```python
from build123d import *

# Parameters (mm, degrees)
BOSS_EXTRUDE1_DEPTH = 4
SKETCH3_R           = 2.1
CUT_EXTRUDE1_DEPTH  = 4
CHAMFER1_SIZE       = 3


with BuildPart() as part:
    # Sketch1 → Boss-Extrude1 (new body)
    with BuildSketch(Plane(origin=(0, 0, 0), x_dir=(1, 0, 0), z_dir=(0, 1, 0))):
        Polygon((0, 0), (0, 80), (20, 80), (80, 20), (80, 0), align=None)
    extrude(amount=BOSS_EXTRUDE1_DEPTH)

    # Sketch3 → Cut-Extrude1 (cut)
    with BuildSketch(Plane(origin=(0, 4, 0), x_dir=(1, 0, 0), z_dir=(0, 1, 0))):
        with Locations((10, 10)):
            Circle(SKETCH3_R)
        with Locations((40, 10)):
            Circle(SKETCH3_R)
        with Locations((70, 10)):
            Circle(SKETCH3_R)
        with Locations((10, 40)):
            Circle(SKETCH3_R)
        with Locations((10, 70)):
            Circle(SKETCH3_R)
    extrude(amount=-CUT_EXTRUDE1_DEPTH, mode=Mode.SUBTRACT)

    # Chamfer1
    chamfer1_edges = [part.edges().sort_by_distance(p)[0] for p in [
        (7.9, 4, -70),
        (7.9, 4, -40),
        (67.9, 4, -10),
        (7.9, 4, -10),
        (37.9, 4, -10),
    ]]
    chamfer(chamfer1_edges, length=CHAMFER1_SIZE)


solid = part.part
```
Check sheet for the modelled part. Datum: model origin and axes. Units: mm. Coordinates: 2 decimals unless noted, no trailing zeros. Order: outer loops, then holes, each group sorted by start corner. A loop starts at its lowest first (then second) coordinate and runs counter-clockwise, first axis right, second up. Notation, with made-up numbers: (55.5, -0.5) -> (100.5, -0.5) arc R18 cw to (100.5, 9.5) -> close; hole circle Ø10 at (64, 47). An arc over 180 degrees is marked (long way). Write each question's results on one line, items separated by ' | '. Start each with the question number.
1) Draft check along Z on faces 1 (the face through (50, 2, -50)), 2 (the face through (7.9, 0.51, -10.09)), 3 (the face through (32, 0, -32)). Enter one of: pulls with the +Z half, pulls with the -Z half, needs draft (parallel to the pull), parting line crosses it, or undercut.
2) Section check C-C (z = -10). Enter the section's corners in (x, y), and give its area (3 significant figures).
3) Section check A-A (x = 10). Enter the section's corners in (y, z), and give its area (3 significant figures).
4) Section check D-D (z = -40). Enter the section's corners in (x, y).
5) Material ranges on line 1 along X through (y, z) = (0.85, -10); line 2 along Z through (x, y) = (10, 0.5); line 3 along Z through (x, y) = (8.5, 0.6), recorded low to high.
6) Section check B-B (y = 3.1). Enter the section's corners in (x, z).
7) Depth check by flat-ended pin: pin 1 (2.5 mm diameter, centred on x = 10, z = -70, fed in from -Y); pin 2 (6.5 mm diameter, centred on x = 70, z = -10, fed in from +Y). Enter the tip coordinate at first touch or a pass-through.
Checked values:
1) face 1: pulls with the -Z half | face 2: undercut | face 3: needs draft
2) outline: (0, 0) -> (7.9, 0) -> (7.9, 1) -> (4.9, 4) -> (0, 4) -> close; (12.1, 0) -> (37.9, 0) -> (37.9, 1) -> (34.9, 4) -> (15.1, 4) -> (12.1, 1) -> close; (42.1, 0) -> (67.9, 0) -> (67.9, 1) -> (64.9, 4) -> (45.1, 4) -> (42.1, 1) -> close; (72.1, 0) -> (80, 0) -> (80, 4) -> (75.1, 4) -> (72.1, 1) -> close | area: 243 mm²
3) outline: (0, -80) -> (4, -80) -> (4, -75.1) -> (1, -72.1) -> (0, -72.1) -> close; (0, -67.9) -> (1, -67.9) -> (4, -64.9) -> (4, -45.1) -> (1, -42.1) -> (0, -42.1) -> close; (0, -37.9) -> (1, -37.9) -> (4, -34.9) -> (4, -15.1) -> (1, -12.1) -> (0, -12.1) -> close; (0, -7.9) -> (1, -7.9) -> (4, -4.9) -> (4, 0) -> (0, 0) -> close | area: 243 mm²
4) outline: (0, 0) -> (7.9, 0) -> (7.9, 1) -> (4.9, 4) -> (0, 4) -> close; (12.1, 0) -> (60, 0) -> (60, 4) -> (15.1, 4) -> (12.1, 1) -> close
5) line 1: 0 to 7.9, 12.1 to 37.9, 42.1 to 67.9, 72.1 to 80 | line 2: -80 to -72.1, -67.9 to -42.1, -37.9 to -12.1, -7.9 to 0 | line 3: -80 to -71.47, -68.53 to -41.47, -38.53 to -11.47, -8.53 to 0
6) outline: (0, -80) -> (20, -80) -> (80, -20) -> (80, 0) -> (0, 0) -> close; hole circle Ø8.4 at (10, -70); hole circle Ø8.4 at (10, -40); hole circle Ø8.4 at (10, -10); hole circle Ø8.4 at (40, -10); hole circle Ø8.4 at (70, -10)
7) pin 1: through | pin 2: y = 2.15
